Can you work these out from the drawing? Everything is in mm from the part's minimum corner. A direction names the side the tool comes from. Give positions to 0.01 mm unless a question says otherwise; leave off trailing zeros. Write each loop counter-clockwise with the first axis right and the second up, starting at its lowest first coordinate (ties: lowest second). Pieces come first, ordered by that corner, then holes. Notation, with made-up numbers: (38.5, -22.5) - (95.5, -22.5) arc R18 ccw to (95.5, -2.5) - close; hole circle Ø8 at (16, 21). An arc over 180 degrees is marked (long way). Use a Markdown table: item, result.
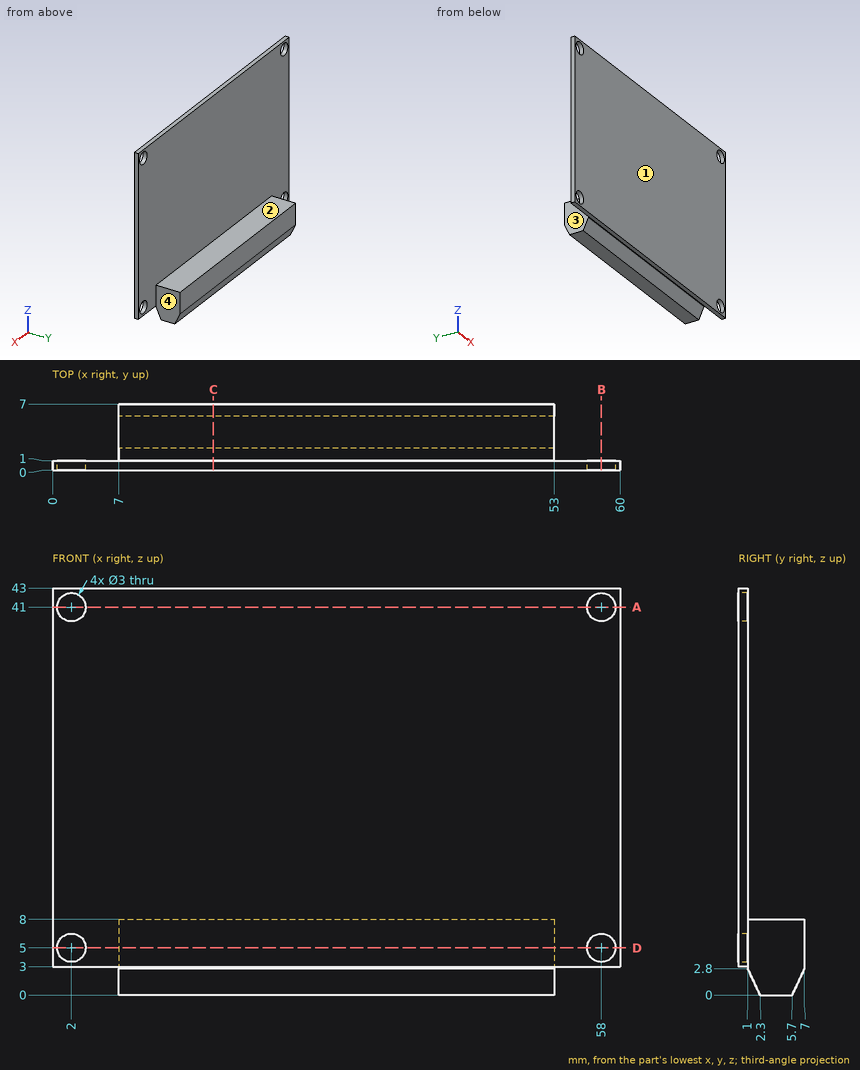
Item 1: If we section it at D-D, the plane z = 5: Write out the boundary of the cut face in (x, y), plus the area to 3 significant figures.
Values:
| item | result |
|---|---|
| outline | (0, 0) - (0.5, 0) - (0.5, 1) - (0, 1) - close; (3.5, 0) - (56.5, 0) - (56.5, 1) - (53, 1) - (53, 7) - (7, 7) - (7, 1) - (3.5, 1) - close; (59.5, 0) - (60, 0) - (60, 1) - (59.5, 1) - close |
| area | 330 mm2 |
Item 2: Will these pins go through, and if not, where does the flat tip stop? pin 1 Ø2 at (x, y) = (19.5, 1) entering from -Z; pin 2 Ø1.8 at (y, z) = (5, 5) entering from -X; pin 3 Ø1 at (x, y) = (23.5, 1) entering from -Z.
Values:
| item | result |
|---|---|
| pin 1 | stops at z = 0.65 |
| pin 2 | stops at x = 7 |
| pin 3 | stops at z = 1.72 |
Item 3: If we section it at B-B, the plane x = 58: Write out the boundary of the cut face in (y, z), plus the area to 3 significant figures.
Values:
| item | result |
|---|---|
| outline | (0, 3) - (1, 3) - (1, 3.5) - (0, 3.5) - close; (0, 6.5) - (1, 6.5) - (1, 39.5) - (0, 39.5) - close; (0, 42.5) - (1, 42.5) - (1, 43) - (0, 43) - close |
| area | 34.0 mm2 |
Item 4: I need wall thicknesses on line 1 along X through (y, z) = (0.45, 5); line 2 along Y through (x, z) = (26, 12); line 3 along Z through (x, y) = (46, 4.75). Which ranges of each line are inside material? Lowest first, please. Write a range as [from, to].
Values:
| item | result |
|---|---|
| line 1 | x = [0, 0.5], [3.5, 56.5], [59.5, 60] |
| line 2 | y = [0, 1] |
| line 3 | z = [0, 8] |
Item 5: If we section it at A-A, the plane z = 41: Write out the boundary of the cut face in (x, y).
Values:
| item | result |
|---|---|
| outline | (0, 0) - (0.5, 0) - (0.5, 1) - (0, 1) - close; (3.5, 0) - (56.5, 0) - (56.5, 1) - (3.5, 1) - close; (59.5, 0) - (60, 0) - (60, 1) - (59.5, 1) - close |
Item 6: For the marked faces 1, 2, 3 and 4, which set-ups out of +Z, -Z, +X, -X, +Y, -Y let a thin tool reach every point of the face, with its end or its side?
Values:
| item | result |
|---|---|
| face 1 | +Z, -Z, +X, -X, -Y |
| face 2 | +Z, +X, -X, +Y |
| face 3 | +Z, -Z, -X, +Y |
| face 4 | +Z, -Z, +X, +Y |
Item 7: If we section it at C-C, the plane x = 17: Write out the boundary of the cut face in (y, z).
Values:
| item | result |
|---|---|
| outline | (0, 3) - (1, 3) - (1, 2.8) - (2.3, 0) - (5.7, 0) - (7, 2.8) - (7, 8) - (1, 8) - (1, 43) - (0, 43) - close |
